CAD build for the part. Positions are in the model's coordinates, mm. Face numbers are marked on the shaded views. A direction names the side the tool comes from. Coordinates: 2 decimals unless noted, no trailing zeros. Order: outer loops, then holes, each group sorted by start corner. A loop starts at its lowest first (then second) coordinate and runs counter-clockwise, first axis right, second up. Notation, with made-up numbers: (6.25, 61.25) - (56.25, 61.25) arc R30 cw to (56.25, 90.25) - close; hole circle Ø3 at (17.5, -29). An arc over 180 degrees is marked (long way). Write each question's results on one line, items separated by ' | '. Start each with the question number.
Q1. Band-saw the part on B-B, the plane z = -16.5. Write the cut outline in (x, y).
Q2. Wall check: probe 1 along X at (y, z) = (12, -15.5); probe 2 along Z at (x, y) = (7.5, 14.25); probe 3 along Z at (x, y) = (21.5, 11.25). Give the ranges that are in metal, low to high.
Q3. Pin check, flat tips, straight feed: P1, Ø10.5, axis at x = 8, z = -15.5, coming from the +Y side; P2, Ø1, axis at x = 2.5, y = 8, coming from the +Z side; P3, Ø3.5, axis at y = 4, z = 9, coming from the +X side. Stop position of each tip, or through.
Q4. Pull direction X, two halves, no side cores. Call the marked faces 1, 2 and 3: released by +X, released by -X, zero draft, split by the parting line, or undercut.
Q5. Which spindle directions (+Z, -Z, +X, -X, +Y, -Y) get a long thin tool onto all of the face, cutting with end or side? Do the marked faces 4 and 5. Say none if no direction does.
Q6. Band-saw the part on C-C, the plane y = 5.25. Write the cut outline in (x, z).
Q7. Band-saw the part on A-A, the plane y = 12.25. Write the cut outline in (x, z), then the cut area to 3 significant figures.
Q8. Band-saw the part on D-D, the plane z = 4. Write the cut outline in (x, y).
```python
from build123d import *

# Parameters (mm, degrees)
SKETCH1_W           = 24.80083823
SKETCH1_H           = 24.80083823
SKETCH1_W_2         = 20.80083823
SKETCH1_H_2         = 20.80083823
EXTRUDE_THIN1_DEPTH = 20.80083823
SKETCH2_W           = 24.80083823
SKETCH2_H           = 24.80083823
BOSS_EXTRUDE1_DEPTH = 2
BOSS_EXTRUDE2_DEPTH = 2
BOSS_EXTRUDE3_DEPTH = 1
FILLET2_R           = 3
EXTRUDE_THIN2_DEPTH = 2
FILLET3_R           = 1


with BuildPart() as part:
    # Sketch1 → Extrude-Thin1 (new body)
    with BuildSketch(Plane(origin=(0, 0, 0), x_dir=(1, 0, 0), z_dir=(0, 1, 0))):
        with Locations((10.400419115, 10.400419115)):
            Rectangle(SKETCH1_W, SKETCH1_H)
        with Locations((10.400419115, 10.400419115)):
            Rectangle(SKETCH1_W_2, SKETCH1_H_2, mode=Mode.SUBTRACT)
    extrude(amount=EXTRUDE_THIN1_DEPTH)

    # Sketch2 → Boss-Extrude1 (add)
    with BuildSketch(Plane.XZ):
        with Locations((10.400419115, -10.400419115)):
            Rectangle(SKETCH2_W, SKETCH2_H)
    extrude(amount=BOSS_EXTRUDE1_DEPTH)

    # Sketch4 → Boss-Extrude2 (add)
    with BuildSketch(Plane.XZ.offset(2)):
        with BuildLine():
            Line((1.884963608, 2), (1.884963608, 28.980417336))
            ThreePointArc((1.884963608, 28.980417336), (10.400419115, 37.495872843), (18.915874622, 28.980417336))
            Line((18.915874622, 28.980417336), (18.915874622, 2))
            ThreePointArc((18.915874622, 2), (10.400419115, -6.515455507), (1.884963608, 2))
        make_face()
    extrude(amount=-BOSS_EXTRUDE2_DEPTH)

    # Sketch5 → Boss-Extrude3 (add, symmetric)
    with BuildSketch(Plane(origin=(10.400419115, 0, 0), x_dir=(0, 0, -1), z_dir=(1, 0, 0))):
        Polygon((-2, 9.400419115), (-15.490208668, 0), (-2, 0), align=None)
    extrude(amount=BOSS_EXTRUDE3_DEPTH, both=True)

    # Fillet2
    fillet2_edges = [part.edges().sort_by_distance(p)[0] for p in [
        (9.400419115, 4.700209558, 2),
        (11.400419115, 4.700209558, 2),
    ]]
    fillet(fillet2_edges, radius=FILLET2_R)

    # Sketch6 → Extrude-Thin2 (add)
    with BuildSketch(Plane(origin=(0, 0, 0), x_dir=(1, 0, 0), z_dir=(0, 1, 0))):
        with BuildLine():
            ThreePointArc((1.884963608, -28.980417336), (10.400419115, -37.495872843), (18.915874622, -28.980417336))
            Line((18.915874622, -28.980417336), (13.915874622, -28.980417336))
            ThreePointArc((13.915874622, -28.980417336), (10.400419115, -32.495872843), (6.884963608, -28.980417336))
            Line((6.884963608, -28.980417336), (1.884963608, -28.980417336))
        make_face()
    extrude(amount=EXTRUDE_THIN2_DEPTH)

    # Fillet3
    fillet3_edges = [part.edges().sort_by_distance(p)[0] for p in [
        (16.415874622, 0, 28.980417336),
        (4.384963608, 0, 28.980417336),
        (10.400419115, 2, 37.495872843),
        (10.400419115, 2, 32.495872843),
        (10.400419115, 0, 32.495872843),
    ]]
    fillet(fillet3_edges, radius=FILLET3_R - 0.0001)  # a hair under: the kernel refuses the full size


solid = part.part
```
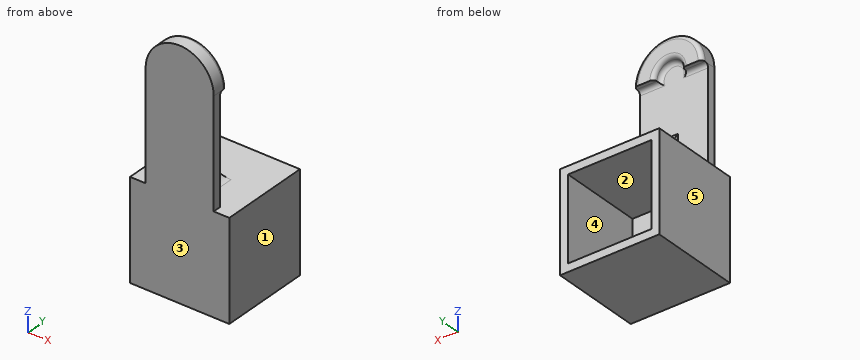
Results below:
1) outline: (-2, -2) - (22.8, -2) - (22.8, 20.8) - (20.8, 20.8) - (20.8, 0) - (0, 0) - (0, 20.8) - (-2, 20.8) - close
2) probe 1: x = -2 to 0, 20.8 to 22.8 | probe 2: z = -22.8 to -20.8, 0 to 2 | probe 3: z = -22.8 to 2
3) P1: stops at y = 0 | P2: stops at z = 2 | P3: stops at x = 11.4
4) face 1: released by +X | face 2: undercut | face 3: zero draft
5) face 4: +Y | face 5: +Z, -Z, -X, +Y, -Y
6) outline: (-2, -22.8) - (22.8, -22.8) - (22.8, 2) - (14.4, 2) arc R3 cw to (11.4, 5) - (11.4, 7.96) - (9.4, 7.96) - (9.4, 5) arc R3 cw to (6.4, 2) - (-2, 2) - close; hole (0, -20.8) - (20.8, -20.8) - (20.8, 0) - (0, 0) - close
7) outline: (-2, -22.8) - (22.8, -22.8) - (22.8, 2) - (-2, 2) - close; hole (0, -20.8) - (20.8, -20.8) - (20.8, 0) - (0, 0) - close | area: 182 mm²
8) outline: (1.88, -2) - (18.92, -2) - (18.92, 0) - (11.57, 0) - (11.57, 8.01) - (9.23, 8.01) - (9.23, 0) - (1.88, 0) - close
